from build123d import *

# Parameters (mm, degrees)
SKETCH1_W               = 89.408
SKETCH1_H               = 48.26
SKETCH1_W_2             = 81.788
SKETCH1_H_2             = 41.656
BOSS_EXTRUDE1_DEPTH     = 127
CUT_EXTRUDE1_DEPTH      = 137.783421934
CUT_EXTRUDE1_DEPTH_BACK = 137.783421934
SKETCH3_R               = 3.429
SKETCH5_W               = 89.408
SKETCH5_H               = 127
SKETCH5_R               = 9.525
BOSS_EXTRUDE3_DEPTH     = 1.905
FILLET1_R               = 0.762


with BuildPart() as part:
    # Sketch1 → Boss-Extrude1 (new body)
    with BuildSketch(Plane(origin=(0, 0, 0), x_dir=(1, 0, 0), z_dir=(0, 1, 0))):
        Rectangle(SKETCH1_W, SKETCH1_H)
        Rectangle(SKETCH1_W_2, SKETCH1_H_2, mode=Mode.SUBTRACT)
    extrude(amount=BOSS_EXTRUDE1_DEPTH)

    # Sketch3 → Cut-Extrude1 (cut, two sides: drawn at the far end of the back side and taken through both)
    with BuildSketch(Plane.XY.offset(-CUT_EXTRUDE1_DEPTH_BACK)):
        with Locations((-18.542, 114.3)):
            Circle(SKETCH3_R)
        with Locations((-18.542, 82.55)):
            Circle(SKETCH3_R)
        with Locations(Location((18.542, 82.55, 0), (0, 0, 180))):
            Circle(SKETCH3_R)
        with Locations(Location((18.542, 114.3, 0), (0, 0, 180))):
            Circle(SKETCH3_R)
        with Locations((18.542, 12.7)):
            Circle(SKETCH3_R)
        with Locations((18.542, 44.45)):
            Circle(SKETCH3_R)
        with Locations(Location((-18.542, 44.45, 0), (0, 0, 180))):
            Circle(SKETCH3_R)
        with Locations(Location((-18.542, 12.7, 0), (0, 0, 180))):
            Circle(SKETCH3_R)
    extrude(amount=CUT_EXTRUDE1_DEPTH + CUT_EXTRUDE1_DEPTH_BACK, mode=Mode.SUBTRACT)

    # Sketch5 → Boss-Extrude3 (add)
    with BuildSketch(Plane(origin=(0, 0, -24.13), x_dir=(-1, 0, 0), z_dir=(0, 0, -1))):
        with Locations((0, 63.5)):
            Rectangle(SKETCH5_W, SKETCH5_H)
        with Locations(Location((18.542, 12.7, 0), (0, 0, 180))):
            Circle(SKETCH5_R, mode=Mode.SUBTRACT)
        with Locations(Location((-18.542, 12.7, 0), (0, 0, 180))):
            Circle(SKETCH5_R, mode=Mode.SUBTRACT)
        with Locations(Location((-18.542, 44.45, 0), (0, 0, 180))):
            Circle(SKETCH5_R, mode=Mode.SUBTRACT)
        with Locations(Location((18.542, 44.45, 0), (0, 0, 180))):
            Circle(SKETCH5_R, mode=Mode.SUBTRACT)
        with Locations(Location((18.542, 82.55, 0), (0, 0, 180))):
            Circle(SKETCH5_R, mode=Mode.SUBTRACT)
        with Locations(Location((-18.542, 82.55, 0), (0, 0, 180))):
            Circle(SKETCH5_R, mode=Mode.SUBTRACT)
        with Locations(Location((18.542, 114.3, 0), (0, 0, 180))):
            Circle(SKETCH5_R, mode=Mode.SUBTRACT)
        with Locations(Location((-18.542, 114.3, 0), (0, 0, 180))):
            Circle(SKETCH5_R, mode=Mode.SUBTRACT)
    boss_extrude3 = extrude(amount=BOSS_EXTRUDE3_DEPTH)

    # Mirror3: Boss-Extrude3 across plane
    add(boss_extrude3.mirror(Plane.XY))

    # Fillet1
    fillet1_edges = [part.edges().sort_by_distance(p)[0] for p in [
        (44.704, 63.5, -26.035),
        (-44.704, 63.5, -26.035),
        (44.704, 63.5, 26.035),
        (-44.704, 63.5, 26.035),
        (40.894, 63.5, 20.828),
        (40.894, 63.5, -20.828),
        (-40.894, 63.5, -20.828),
        (-40.894, 63.5, 20.828),
    ]]
    fillet(fillet1_edges, radius=FILLET1_R)


solid = part.part
Work out the finished part from the listing and answer in its coordinate system (mm). A direction names the side the tool comes from. Give positions to 0.01 mm unless a question says otherwise; leave off trailing zeros. Loops run counter-clockwise (first coordinate to the right, second up) from the corner with the lowest first, then second, coordinate; pieces in that order, holes last. Notation, with made-up numbers: (37.5, 27.25) -> (58.5, 27.25) arc R35 ccw to (58.5, 63.25) -> close; hole circle Ø4 at (80.5, 68). An arc over 180 degrees is marked (long way). Use a Markdown table: item, result. Add a question column.
1. Find the intervals of material crossed by probe 1 along X at (y, z) = (114, -22); probe 2 along X at (y, z) = (44, -22.5); probe 3 along X at (y, z) = (38, -8.5), in increasing order.
2. Section C-C on y = 59 is taken. Determine the outline of the cut face in (x, z) (3 decimals).
3. Section A-A on x = 4.5 is taken. Determine the outline of the cut face in (y, z) (3 decimals).
4. Determine the mould class of faces 4 (the cylindrical face through (-19.285, 79.203, 22.456)), 5 (the flat face through (-1, 63, 20.828)), 6 (the flat face through (-14, 44, 24.13)), 7 (the flat face through (23, 13, -24.13)) for opening direction Z: released by +Z, released by -Z, zero draft, split by the parting line, or undercut.
5. Section D-D on y = 44.45 is taken. State how many separate pieces and enclosed holes the cut face has, and give its area (3 significant figures).
6. Flat-ended cylindrical pins translate along their axes: pin 1 Ø11.5 at (x, y) = (18.542, 44.45) entering from -Z; pin 2 Ø9 at (x, y) = (-18.542, 44.45) entering from +Z. Find the tip coordinate at first contact, or state that the pin passes through.
7. Section B-B on z = 2.5 is taken. Determine the outline of the cut face in (x, y), and give its area (3 significant figures).
8. For faces 1 (the flat face through (-14, 82, 24.13)), 2 (the cylindrical face through (16.7, 111.41, 22.46)), 3 (the cylindrical face through (-28.058, 12.281, -25.069)), determine the directions among +Z, -Z, +X, -X, +Y, -Y from which every point of the face is accessible in a straight line to the end or side of a thin tool.
Results below:
| question | item | result |
|---|---|---|
| 1 | probe 1 | x = -44.7 to -21.96, -15.13 to 15.13, 21.96 to 44.7 |
| 1 | probe 2 | x = -44.7 to -21.94, -15.14 to 15.14, 21.94 to 44.7 |
| 1 | probe 3 | x = -44.7 to -40.89, 40.89 to 44.7 |
| 2 | outline | (-44.704, -25.273) arc R0.762 ccw to (-43.942, -26.035) -> (43.942, -26.035) arc R0.762 ccw to (44.704, -25.273) -> (44.704, 25.273) arc R0.762 ccw to (43.942, 26.035) -> (-43.942, 26.035) arc R0.762 ccw to (-44.704, 25.273) -> close; hole (-40.894, -20.066) arc R0.762 ccw to (-40.132, -20.828) -> (40.132, -20.828) arc R0.762 ccw to (40.894, -20.066) -> (40.894, 20.066) arc R0.762 ccw to (40.132, 20.828) -> (-40.132, 20.828) arc R0.762 ccw to (-40.894, 20.066) -> close |
| 3 | outline | (0, -26.035) -> (127, -26.035) -> (127, -20.828) -> (0, -20.828) -> close; (0, 20.828) -> (127, 20.828) -> (127, 26.035) -> (0, 26.035) -> close |
| 4 | face 4 | zero draft |
| 4 | face 5 | undercut |
| 4 | face 6 | released by +Z |
| 4 | face 7 | released by -Z |
| 5 | separate pieces | 4 |
| 5 | enclosed holes | 0 |
| 5 | area | 1,010 mm^2 |
| 6 | pin 1 | stops at z = -24.13 |
| 6 | pin 2 | stops at z = 24.13 |
| 7 | outline | (-44.7, 0) -> (-40.89, 0) -> (-40.89, 127) -> (-44.7, 127) -> close; (40.89, 0) -> (44.7, 0) -> (44.7, 127) -> (40.89, 127) -> close |
| 7 | area | 968 mm^2 |
| 8 | face 1 | +Z |
| 8 | face 2 | +Z, -Z |
| 8 | face 3 | -Z |
